```python
from build123d import *

# Parameters (mm, degrees)
F1_DEPTH  = 28
F2_R      = 5
F3_DEPTH  = 5.001
F4_R      = 3.5
F5_DEPTH  = 44.7891304684
F7_DEPTH  = 5
F9_DEPTH  = 5
F11_DEPTH = 5.24
F13_DEPTH = 5.24


with BuildPart() as f1:
    # F0 (on Top) → F1 (new body)
    with BuildSketch(Plane.XY):
        Polygon((52.8867513459, 5), (0, 5), (0, 0), (50, 0), (94.5, -77.0762609368), (98.8301270189, -74.5762609368), align=None)
    extrude(amount=F1_DEPTH)

    # F2 (on face) → F3 (cut, through all)
    with BuildSketch(Plane.XZ):
        with Locations((25, 14)):
            Circle(F2_R)
    extrude(amount=-F3_DEPTH, mode=Mode.SUBTRACT)

    # F4 (on face) → F5 (cut, through all)
    with BuildSketch(Plane(origin=(37.5, 21.6506350946, 0), x_dir=(0.5, -0.8660254038, 0), z_dir=(-0.8660254038, -0.5, 0))):
        with Locations((76.5, 14)):
            Circle(F4_R)
    extrude(amount=-F5_DEPTH, mode=Mode.SUBTRACT)

    # F6 (on Top) → F7 (join)
    with BuildSketch(Plane.XY):
        Polygon((50, 0), (20, 0), (65, -25.9807621135), align=None)
    extrude(amount=F7_DEPTH)

    # F8 (on face) → F9 (join)
    with BuildSketch(Plane.XY.offset(28)):
        Polygon((65, -25.9807621135), (50, 0), (20, 0), align=None)
    extrude(amount=-F9_DEPTH)

    # F10 (on face) → F11 (join)
    with BuildSketch(Plane(origin=(41.8301270189, 24.1506350946, 0), x_dir=(-0.5, 0.8660254038, 0), z_dir=(0.8660254038, 0.5, 0))):
        Polygon((-85.0626, 18.943619415), (-85.0626, 9.056380585), (-76.5, 4.1127611701), (-67.9374, 9.056380585), (-67.9374, 18.943619415), (-76.5, 23.8872388299), align=None)
        Polygon((-76.5, 20.4231372148), (-70.9374, 17.2115686074), (-70.9374, 10.7884313926), (-76.5, 7.5768627852), (-82.0626, 10.7884313926), (-82.0626, 17.2115686074), align=None, mode=Mode.SUBTRACT)
    extrude(amount=F11_DEPTH)

    # F12 (on face) → F13 (join, through all)
    with BuildSketch(Plane(origin=(41.8301270189, 24.1506350946, 0), x_dir=(-0.5, 0.8660254038, 0), z_dir=(0.8660254038, 0.5, 0))):
        Polygon((-75.5, 0), (-75.5, 4.6901114393), (-76.5, 4.1127611701), (-77.5, 4.6901114393), (-77.5, 0), align=None)
    extrude(amount=F13_DEPTH)


solid = f1.part
```
Could you check a few things on this model? Use its own coordinates, in mm. A direction names the side the tool comes from. Round coordinates to 2 decimals unless told otherwise and drop trailing zeros. Write each loop counter-clockwise with the first axis right and the second up, starting at its lowest first coordinate (ties: lowest second). Pieces come first, ordered by that corner, then holes. Notation, with made-up numbers: M 46,62.5 L 67,62.5 A23 ccw 67,87.5 Z; hole C 39,64 d9. An arc over 180 degrees is marked long. Write each question's results on one line, items separated by ' | '. Start each with the question number.
1. On a 3-axis mill with a long thin cutter (end or side, diameter ignored), from which of +Z, -Z, +X, -X, +Y, -Y can I reach the whole of each face in a straight line? I mean faces 1 (the face through (81.82, -39.94, 2.31)), 2 (the face through (44, -8, 23)), 3 (the face through (54, -17, 0)), 4 (the face through (82.817, -41.675, 2.378)), 5 (the face through (83.727, -43.251, 18.795)). Say none if no direction works.
2. I need wall thicknesses on L1, parallel to Z at x = 25, y = 2.6; L2, parallel to Z at x = 53, y = -9.5; L3, parallel to Y at x = 12, z = 20.75. Which ranges of each line are inside material? Lowest first, please. Write a range as from..to.
3. I'm going to push flat-ended pins straight in: pin 1 Ø10 at (y, z) = (-57, 8.5) entering from +X; pin 2 Ø10 at (x, y) = (80, -22) entering from -Z; pin 3 Ø5 at (x, y) = (81.5, -35) entering from -Z; pin 4 Ø10 at (y, z) = (-27.5, 19.5) entering from -X. Where does each tip first touch, or does it pass through?
4. Imagine slicing it at C-C on x = 59.5. List the corners of the cut face in (y, z) for me, and give its area (3 significant figures).
5. Imagine slicing it at D-D on y = -12. List the corners of the cut face in (x, z) for me.
6. Imagine slicing it at B-B on z = 14. List the corners of the cut face in (x, y) for me.
7. Imagine slicing it at A-A on x = 25. List the corners of the cut face in (y, z) for me.
8. Thinking about a two-plate mould opening in Y: for faces 6 (the face through (79.953, -36.714, 6.843)), 7 (the face through (83.69, -43.18, 9.16)), 8 (the face through (53, -15, 28)), 9 (the face through (76.5, -40.96, 11.87)), which applies, +Y half, -Y half, draft (parallel to the pull), parting line (faces both ways), or undercut?
Result sheet:
1) face 1: -Z, +Y | face 2: -X, -Y | face 3: -Z, +X, -X, +Y, -Y | face 4: -Z, +X | face 5: none
2) L1: z = 0..9, 19..28 | L2: z = 0..5, 23..28 | L3: y = 0..5
3) pin 1: stops at x = 91.57 | pin 2: passes through | pin 3: stops at z = 5.81 | pin 4: stops at x = 61.45
4) outline: M -22.81,0 L -6.45,0 L -6.45,28 L -22.81,28 L -22.81,23 L -16.45,23 L -16.45,5 L -22.81,5 Z | area: 344 mm^2
5) outline: M 40.78,0 L 62.7,0 L 62.7,28 L 40.78,28 L 40.78,23 L 56.93,23 L 56.93,5 L 40.78,5 Z
6) outline: M 0,0 L 20,0 L 20,5 L 0,5 Z; M 30,0 L 50,0 L 74,-41.57 L 78.33,-39.07 L 77.3,-37.28 L 81.84,-34.66 L 80.34,-32.06 L 75.8,-34.68 L 52.89,5 L 30,5 Z; M 77.5,-47.63 L 94.5,-77.08 L 98.83,-74.58 L 84.36,-49.52 L 88.9,-46.9 L 87.4,-44.3 L 82.86,-46.92 L 81.83,-45.13 Z
7) outline: M -2.89,0 L 5,0 L 5,9 L 0,9 L 0,5 L -2.89,5 Z; M -2.89,23 L 0,23 L 0,19 L 5,19 L 5,28 L -2.89,28 Z
8) face 6: +Y half | face 7: undercut | face 8: draft | face 9: undercut
